For this review, take the finished solid that the model builds, in its own axes (mm). A direction names the side the tool comes from. Coordinates: 2 decimals unless noted, no trailing zeros. Write each loop counter-clockwise with the first axis right and the second up, starting at its lowest first coordinate (ties: lowest second). Pieces come first, ordered by that corner, then holes.
1) Mouldability with a two-part tool opening along Y and no side actions: class faces 3 (the face through (-17, -38, 40)), 4 (the face through (-40, -1, 39)), 5 (the face through (-1, 40, 39)) as pulls with the +Y half, pulls with the -Y half, needs draft (parallel to the pull), parting line crosses it, or undercut.
2) Insertion check: P1, Ø4, axis at x = 31.5, y = -27, coming from the +Z side. The pin has a flat end and moves straight along its axis. Give the tip position at first contact, or say it passes through.
3) We need section B-B on x = -14. Write out the cut boundary in (y, z).
4) We need section C-C on y = -31.5. Write out the cut boundary in (x, z).
5) To check wall thickness, follow line 1 along X through (y, z) = (-36, 29); line 2 along Y through (x, z) = (14, 65); line 3 along Z through (x, y) = (-32, 10). State the ranges of each line that lie inside material, in increasing order.
6) For faces 1 (the face through (-1, 1, 2)), 2 (the face through (-1, 1, 0)), list the 3-axis set-ups (+Z, -Z, +X, -X, +Y, -Y) from which the entire face can be reached by the end or side of a thin tool; tool diameter is ignored.
7) We need section A-A on z = 17. Write out the cut boundary in (x, y), then the cut area to 3 significant figures.
from build123d import *

# Parameters (mm, degrees)
F0_W     = 80
F0_H     = 80
F0_W_2   = 75.8
F0_H_2   = 76
F1_DEPTH = 80
F2_DEPTH = 2
F4_DEPTH = 25
F5_R     = 1.5


with BuildPart() as f1:
    # F0 (on Top) → F1 (new body)
    with BuildSketch(Plane.XY):
        Rectangle(F0_W, F0_H)
        Rectangle(F0_W_2, F0_H_2, mode=Mode.SUBTRACT)
    extrude(amount=F1_DEPTH)

    # F0 (on Top) → F2 (join)
    with BuildSketch(Plane.XY):
        Rectangle(F0_W_2, F0_H_2)
    extrude(amount=F2_DEPTH)

    # F3 (on face) → F4 (cut)
    with BuildSketch(Plane.XZ.offset(40)):
        with BuildLine():
            Line((0, 40), (0, 60))
            add(Edge.make_bspline(
                [(0, 60), (-12.5, 60), (-12.5, 40)],
                knots=[0, 0, 0, 1.5707963268, 1.5707963268, 1.5707963268], degree=2, weights=[1, 0.7071067812, 1]))
            Line((-12.5, 40), (0, 40))
        make_face()
        with BuildLine():
            add(Edge.make_bspline(
                [(12.5, 40), (12.5, 60), (0, 60)],
                knots=[4.7123889804, 4.7123889804, 4.7123889804, 6.2831853072, 6.2831853072, 6.2831853072], degree=2, weights=[1, 0.7071067812, 1]))
            Line((0, 60), (0, 40))
            Line((0, 40), (12.5, 40))
        make_face()
        with BuildLine():
            Line((12.5, 40), (0, 40))
            Line((0, 40), (0, 20))
            add(Edge.make_bspline(
                [(0, 20), (12.5, 20), (12.5, 40)],
                knots=[3.1415926536, 3.1415926536, 3.1415926536, 4.7123889804, 4.7123889804, 4.7123889804], degree=2, weights=[1, 0.7071067812, 1]))
        make_face()
        with BuildLine():
            Line((0, 20), (0, 40))
            Line((0, 40), (-12.5, 40))
            add(Edge.make_bspline(
                [(-12.5, 40), (-12.5, 20), (0, 20)],
                knots=[1.5707963268, 1.5707963268, 1.5707963268, 3.1415926536, 3.1415926536, 3.1415926536], degree=2, weights=[1, 0.7071067812, 1]))
        make_face()
    extrude(amount=-F4_DEPTH, mode=Mode.SUBTRACT)

    # F5
    f5_edges = [f1.edges().sort_by_distance(p)[0] for p in [
        (-40, -40, 40),
        (40, 40, 40),
        (-40, 40, 40),
        (40, -40, 40),
    ]]
    fillet(f5_edges, radius=F5_R)


solid = f1.part
Result:
1. face 3: undercut
1. face 4: needs draft
1. face 5: pulls with the +Y half
2. P1: stops at z = 2
3. outline: (-40, 0) - (40, 0) - (40, 80) - (38, 80) - (38, 2) - (-38, 2) - (-38, 80) - (-40, 80) - close
4. outline: (-40, 0) - (40, 0) - (40, 80) - (37.9, 80) - (37.9, 2) - (-37.9, 2) - (-37.9, 80) - (-40, 80) - close
5. line 1: x = -40 to -37.9, 37.9 to 40
5. line 2: y = -40 to -38, 38 to 40
5. line 3: z = 0 to 2
6. face 1: +Z
6. face 2: -Z, +X, -X, +Y, -Y
7. outline: (-40, -38.5) arc R1.5 ccw to (-38.5, -40) - (38.5, -40) arc R1.5 ccw to (40, -38.5) - (40, 38.5) arc R1.5 ccw to (38.5, 40) - (-38.5, 40) arc R1.5 ccw to (-40, 38.5) - close; hole (-37.9, -38) - (37.9, -38) - (37.9, 38) - (-37.9, 38) - close
7. area: 637 mm2
